For this review, use the dimensioned drawing (mm, ordinates from the lowest corner) and the shaded views. Coordinates: 2 decimals unless noted, no trailing zeros. Write each loop counter-clockwise with the first axis right and the second up, starting at its lowest first coordinate (ties: lowest second). Pieces come first, ordered by that corner, then holes. Notation, with made-up numbers: (28, 42) -> (75, 42) arc R17 ccw to (75, 48) -> close; hole circle Ø2 at (39, 59). An arc over 180 degrees is marked (long way). Put each result on its own line as item: value. Start each with the question number.
Item 1: The part is to be moulded in two halves that separate along Y. For the marked faces 1, 2, 3 and 4, say which applies: +Y half, -Y half, draft (parallel to the pull), parting line (faces both ways), or undercut.
Item 2: Consider section B-B on z = 7.5. Give the number of separate pieces and of enclosed holes in the cut face.
Item 3: Consider section A-A on y = 9. Give the boundary of the cut face in (x, z).
Item 4: To check wall thickness, follow L1, parallel to Z at x = 12, y = 8; L2, parallel to X at y = 27, z = 15.5; L3, parallel to Y at x = 9.75, z = 6.35. State the ranges of each line that lie inside material, in increasing order.
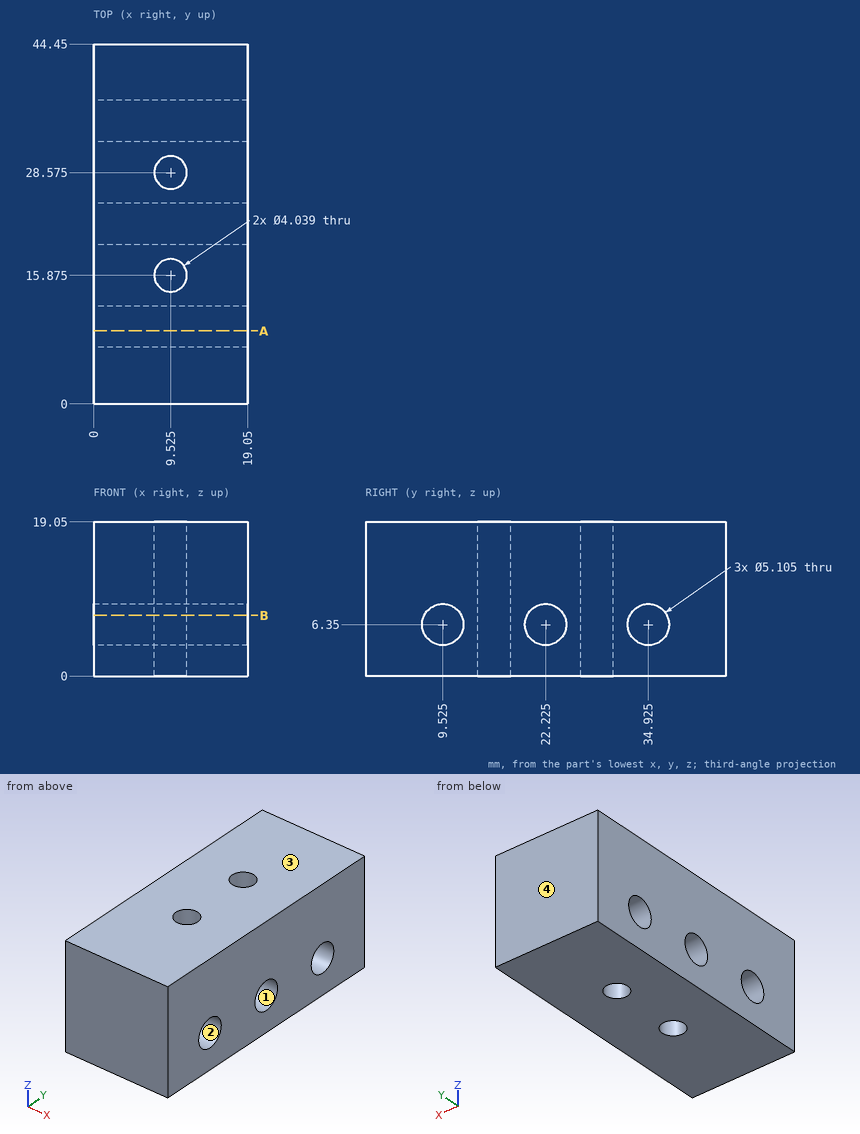
Return value:
1. face 1: undercut
1. face 2: undercut
1. face 3: draft
1. face 4: +Y half
2. separate pieces: 4
2. enclosed holes: 2
3. outline: (0, 0) -> (19.05, 0) -> (19.05, 3.85) -> (0, 3.85) -> close; (0, 8.85) -> (19.05, 8.85) -> (19.05, 19.05) -> (0, 19.05) -> close
4. L1: 0 to 4.3, 8.4 to 19.05
4. L2: 0 to 8.26, 10.79 to 19.05
4. L3: 0 to 6.97, 12.08 to 13.87, 17.88 to 19.67, 24.78 to 26.57, 30.58 to 32.37, 37.48 to 44.45
